For this review, take the finished solid that the model builds, in its own axes (mm). Face numbers are marked on the shaded views. A direction names the side the tool comes from. Give positions to 0.01 mm unless a question says otherwise; leave off trailing zeros. Write each loop counter-clockwise with the first axis right and the second up, starting at its lowest first coordinate (ties: lowest second). Pieces come first, ordered by that corner, then holes. Notation, with made-up numbers: M 65,79.5 L 77,79.5 A22 ccw 77,109.5 Z; hole C -16,0 d5. An arc over 180 degrees is marked long. Use one line per item in the form item = value. Start each with the question number.
Q1. Consider section B-B on x = -20. Write out the cut boundary in (y, z).
Q2. Consider section A-A on z = 8.5. Write out the cut boundary in (x, y).
Q3. For probe 1 along Y at (x, z) = (5.5, 35); probe 2 along X at (y, z) = (-22.5, 30); probe 3 along X at (y, z) = (34.35, 8.5), list the stretches that pass through material, from the lowest coordinate up. Write a range as [from, to].
Q4. Mouldability with a two-part tool opening along Y and no side actions: class the marked faces 1, 2 and 3 as released by +Y, released by -Y, zero draft, split by the parting line, or undercut.
Q5. Consider section C-C on y = -25.5. Write out the cut boundary in (x, z).
Q6. Consider section D-D on x = -49. Write out the cut boundary in (y, z).
Q7. Tool access review of the marked faces 4 and 5: name each direction out of +Z, -Z, +X, -X, +Y, -Y from which nothing blocks a thin tool from reaching the whole face with its end or side.
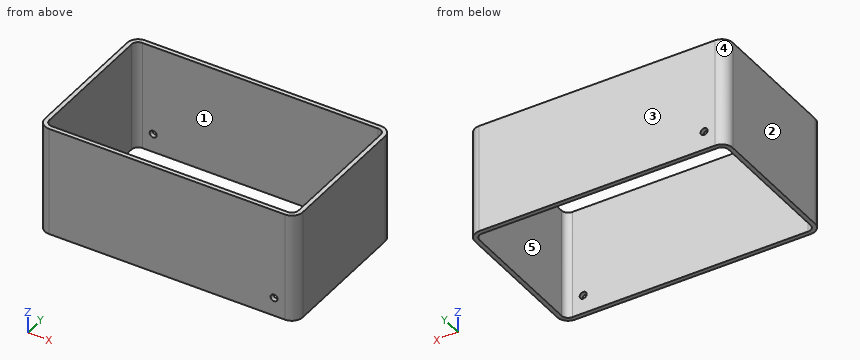
```python
from build123d import *

# Parameters (mm, degrees)
SKETCH_1_W          = 118
SKETCH_1_H          = 70
EXTRUDE_1_DEPTH     = 50
FILLET_1_R          = 5
CUT_EXTRUDE_1_DEPTH = 85.888161719
CUT_EXTRUDE_2_REACH = 106.312
SKETCH_3_R          = 1.6
SKETCH_4_R          = 1.6
CUT_EXTRUDE_3_DEPTH = 50


with BuildPart() as part:
    # ｽｹｯﾁ1 → ﾎﾞｽ - 押し出し1 (new body)
    with BuildSketch(Plane.XY):
        Rectangle(SKETCH_1_W, SKETCH_1_H)
    extrude(amount=EXTRUDE_1_DEPTH)

    # ﾌｨﾚｯﾄ1
    fillet_1_edges = [part.edges().sort_by_distance(p)[0] for p in [
        (59, -35, 25),
        (-59, -35, 25),
        (-59, 35, 25),
        (59, 35, 25),
    ]]
    fillet(fillet_1_edges, radius=FILLET_1_R)

    # ｽｹｯﾁ2 → ｶｯﾄ - 押し出し1 (cut, through all)
    with BuildSketch(Plane.XY.offset(50)):
        with BuildLine():
            Line((-54, -33), (54, -33))
            ThreePointArc((54, -33), (56.121320344, -32.121320344), (57, -30))
            Line((57, -30), (57, 30))
            ThreePointArc((57, 30), (56.121320344, 32.121320344), (54, 33))
            Line((54, 33), (-54, 33))
            ThreePointArc((-54, 33), (-56.121320344, 32.121320344), (-57, 30))
            Line((-57, 30), (-57, -30))
            ThreePointArc((-57, -30), (-56.121320344, -32.121320344), (-54, -33))
        make_face()
    extrude(amount=-CUT_EXTRUDE_1_DEPTH, mode=Mode.SUBTRACT)

    # ｽｹｯﾁ3 → ｶｯﾄ - 押し出し2 (cut, up to next)
    with BuildSketch(Plane.XZ.offset(35), mode=Mode.PRIVATE) as cut_extrude_2_sk1:
        with Locations(Location((49, 8.5, 0), (0, 0, 270))):
            Circle(SKETCH_3_R)
    cut_extrude_2_tool1 = extrude(cut_extrude_2_sk1.sketch, amount=-CUT_EXTRUDE_2_REACH, mode=Mode.PRIVATE) & part.part
    add(cut_extrude_2_tool1.solids().sort_by_distance((49, -35, 8.5))[0], mode=Mode.SUBTRACT)

    # ｽｹｯﾁ4 → ｶｯﾄ - 押し出し3 (cut)
    with BuildSketch(Plane(origin=(0, 35, 0), x_dir=(1, 0, 0), z_dir=(0, 1, 0))):
        with Locations(Location((-49, -8.5, 0), (0, 0, 270))):
            Circle(SKETCH_4_R)
    extrude(amount=-CUT_EXTRUDE_3_DEPTH, mode=Mode.SUBTRACT)


solid = part.part
```
Working result:
q1.outline = M -35,0 L -33,0 L -33,50 L -35,50 Z; M 33,0 L 35,0 L 35,50 L 33,50 Z
q2.outline = M -59,-30 A5 ccw -54,-35 L 47.4,-35 L 47.4,-33 L -54,-33 A3 cw -57,-30 L -57,30 A3 cw -54,33 L -50.6,33 L -50.6,35 L -54,35 A5 ccw -59,30 Z; M -47.4,33 L 54,33 A3 cw 57,30 L 57,-30 A3 cw 54,-33 L 50.6,-33 L 50.6,-35 L 54,-35 A5 ccw 59,-30 L 59,30 A5 ccw 54,35 L -47.4,35 Z
q3.probe_1 = [-35, -33], [33, 35]
q3.probe_2 = [-59, -57], [57, 59]
q3.probe_3 = [-56.47, -50.6], [-47.4, 56.47]
q4.face_1 = undercut
q4.face_2 = zero draft
q4.face_3 = released by +Y
q5.outline = M -59,0 L -57,0 L -57,50 L -59,50 Z; M 57,0 L 59,0 L 59,50 L 57,50 Z
q6.outline = M -35,0 L -33,0 L -33,50 L -35,50 Z; M 33,0 L 35,0 L 35,6.9 L 33,6.9 Z; M 33,10.1 L 35,10.1 L 35,50 L 33,50 Z
q7.face_4 = +Z, -Z, -X, +Y
q7.face_5 = +Z, -Z
